Verification items for the finished model (mm, model axes). A direction names the side the tool comes from. Give positions to 0.01 mm unless a question says otherwise; leave off trailing zeros. Loops run counter-clockwise (first coordinate to the right, second up) from the corner with the lowest first, then second, coordinate; pieces in that order, holes last. Notation, with made-up numbers: (45.25, 65.25) - (64.25, 65.25) arc R16 ccw to (64.25, 95.25) - close; hole circle Ø10 at (82, 29). An arc over 180 degrees is marked (long way). Answer in a Markdown table with one row per item.
```python
from build123d import *

# Parameters (mm, degrees)
CROQUIS1_W              = 96
CROQUIS1_H              = 64
SALIENTE_EXTRUIR1_DEPTH = 70
VACIADO1_T              = -2
CROQUIS2_R              = 16
CORTAR_EXTRUIR1_DEPTH   = 5
CROQUIS3_R              = 19.5
CORTAR_EXTRUIR2_DEPTH   = 5


with BuildPart() as part:
    # Croquis1 → Saliente-Extruir1 (new body)
    with BuildSketch(Plane(origin=(0, 0, 0), x_dir=(1, 0, 0), z_dir=(0, 1, 0))):
        Rectangle(CROQUIS1_W, CROQUIS1_H)
    extrude(amount=SALIENTE_EXTRUIR1_DEPTH)

    # Vaciado1
    vaciado1_openings = [part.faces().sort_by_distance(p)[0] for p in [
        (0, 0, 0),
    ]]
    offset(amount=VACIADO1_T, openings=vaciado1_openings, kind=Kind.INTERSECTION)

    # Croquis2 → Cortar-Extruir1 (cut)
    with BuildSketch(Plane(origin=(0, 70, 0), x_dir=(1, 0, 0), z_dir=(0, 1, 0))):
        Circle(CROQUIS2_R)
    extrude(amount=-CORTAR_EXTRUIR1_DEPTH, mode=Mode.SUBTRACT)

    # Croquis3 → Cortar-Extruir2 (cut)
    with BuildSketch(Plane.XY.offset(32)):
        with Locations((0, 30.5)):
            Circle(CROQUIS3_R)
    extrude(amount=-CORTAR_EXTRUIR2_DEPTH, mode=Mode.SUBTRACT)


solid = part.part
```
Q1. Sectioned sample at D-D (x = -1). Record the cut outline in (y, z).
Completed:
| item | result |
|---|---|
| outline | (0, -32) - (70, -32) - (70, -15.97) - (68, -15.97) - (68, -30) - (0, -30) - close; (0, 30) - (11.03, 30) - (11.03, 32) - (0, 32) - close; (49.97, 30) - (68, 30) - (68, 15.97) - (70, 15.97) - (70, 32) - (49.97, 32) - close |
Q2. Tool access check on faces 4 (the face through (46, 34, 0)), 5 (the face through (-4.227, 11.464, 31.014)), 6 (the face through (-14, 0, -31)). Record the directions out of +Z, -Z, +X, -X, +Y, -Y that give a thin tool (end or side, any length) a straight path to the whole face; none if there is none.
Completed:
| item | result |
|---|---|
| face 4 | -Y |
| face 5 | +Z |
| face 6 | +Z, -Z, +X, -X, -Y |
Q3. Go/stop test with a flat-tipped pin: P1, Ø19, axis at x = 0, z = 0, coming from the -Y side. Record where the tip stops, or that it passes through.
Completed:
| item | result |
|---|---|
| P1 | through |
Q4. Sectioned sample at C-C (x = 18). Record the cut outline in (y, z), and give its area (3 significant figures).
Completed:
| item | result |
|---|---|
| outline | (0, -32) - (70, -32) - (70, 32) - (38, 32) - (38, 30) - (68, 30) - (68, -30) - (0, -30) - close; (0, 30) - (23, 30) - (23, 32) - (0, 32) - close |
| area | 370 mm^2 |
Q5. Sectioned sample at B-B (y = 65). Record the cut outline in (x, z), and give its area (3 significant figures).
Completed:
| item | result |
|---|---|
| outline | (-48, -32) - (48, -32) - (48, 32) - (-48, 32) - close; hole (-46, -30) - (46, -30) - (46, 30) - (-46, 30) - close |
| area | 624 mm^2 |
Q6. Thickness scan on line 1 (X direction, y = 3.5, z = -9.5); line 2 (Z direction, x = 0, y = 69.2); line 3 (Z direction, x = -2.5, y = 4.5). Record the ranges inside material, lowest first.
Completed:
| item | result |
|---|---|
| line 1 | -48 to -46, 46 to 48 |
| line 2 | -32 to -16, 16 to 32 |
| line 3 | -32 to -30, 30 to 32 |
Q7. Draft check along X on faces 1 (the face through (-11, 49, 30)), 2 (the face through (48, 35, 0)), 3 (the face through (-11, 50, 32)). Enter one of: +X half, -X half, draft (parallel to the pull), parting line (faces both ways), or undercut.
Completed:
| item | result |
|---|---|
| face 1 | undercut |
| face 2 | +X half |
| face 3 | draft |
Q8. Sectioned sample at A-A (z = 0). Record the cut outline in (x, y).
Completed:
| item | result |
|---|---|
| outline | (-48, 0) - (-46, 0) - (-46, 68) - (-16, 68) - (-16, 70) - (-48, 70) - close; (16, 68) - (46, 68) - (46, 0) - (48, 0) - (48, 70) - (16, 70) - close |
